```python
from build123d import *

# Parameters (mm, degrees)
F1_DEPTH = 63.5
F2_DEPTH = 25.4
F3_DEPTH = 12.7


with BuildPart() as f1:
    # F0 (on Front) → F1 (new body, symmetric)
    with BuildSketch(Plane.XZ):
        Polygon((41.275, -9.525), (41.275, 9.525), (22.225, 9.525), (-41.275, 9.525), (-41.275, -9.525), align=None)
    extrude(amount=F1_DEPTH, both=True)

    # F0 (on Front) → F2 (join, symmetric)
    with BuildSketch(Plane.XZ):
        with BuildLine():
            Line((22.225, 9.525), (41.275, 9.525))
            Line((41.275, 9.525), (41.275, 27.0002))
            ThreePointArc((41.275, 27.0002), (45.92468, 38.22552), (57.15, 42.8752))
            Line((57.15, 42.8752), (60.325, 42.8752))
            Line((60.325, 42.8752), (60.325, 61.9252))
            Line((60.325, 61.9252), (57.15, 61.9252))
            add(Edge.make_bspline(
                [(47.359648, 60.524887), (50.585981, 60.958071), (53.852213, 61.418514), (57.15, 61.9252)],
                knots=[103.904847, 103.904847, 103.904847, 103.904847, 111.504536, 111.504536, 111.504536, 111.504536], degree=3))
            ThreePointArc((47.359648, 60.524887), (29.206453, 47.950469), (22.225, 27.0002))
            Line((22.225, 27.0002), (22.225, 9.525))
        make_face()
        Polygon((60.325, 61.9252), (60.325, 42.8752), (60.325, 38.1), (111.125, 38.1), (111.125, 66.675), (60.325, 66.675), align=None)
    extrude(amount=F2_DEPTH, both=True)

    # F0 (on Front) → F3 (join, symmetric)
    with BuildSketch(Plane.XZ):
        Polygon((41.275, -9.525), (41.275, 9.525), (22.225, 9.525), (-41.275, 9.525), (-41.275, -9.525), align=None)
        with BuildLine():
            Line((22.225, 9.525), (41.275, 9.525))
            Line((41.275, 9.525), (41.275, 27.0002))
            ThreePointArc((41.275, 27.0002), (45.92468, 38.22552), (57.15, 42.8752))
            Line((57.15, 42.8752), (60.325, 42.8752))
            Line((60.325, 42.8752), (60.325, 61.9252))
            Line((60.325, 61.9252), (57.15, 61.9252))
            add(Edge.make_bspline(
                [(47.359648, 60.524887), (50.585981, 60.958071), (53.852213, 61.418514), (57.15, 61.9252)],
                knots=[103.904847, 103.904847, 103.904847, 103.904847, 111.504536, 111.504536, 111.504536, 111.504536], degree=3))
            ThreePointArc((47.359648, 60.524887), (29.206453, 47.950469), (22.225, 27.0002))
            Line((22.225, 27.0002), (22.225, 9.525))
        make_face()
        with BuildLine():
            Line((-41.275, 9.525), (22.225, 9.525))
            Line((22.225, 9.525), (22.225, 27.0002))
            ThreePointArc((22.225, 27.0002), (29.206453, 47.950469), (47.359648, 60.524887))
            add(Edge.make_bspline(
                [(-41.275, 9.525), (-33.40458, 53.775256), (3.24841, 54.602289), (47.359648, 60.524887)],
                knots=[0, 0, 0, 0, 103.904847, 103.904847, 103.904847, 103.904847], degree=3))
        make_face()
        with BuildLine():
            ThreePointArc((57.15, 61.9252), (52.205006, 61.573349), (47.359648, 60.524887))
            add(Edge.make_bspline(
                [(47.359648, 60.524887), (50.585981, 60.958071), (53.852213, 61.418514), (57.15, 61.9252)],
                knots=[103.904847, 103.904847, 103.904847, 103.904847, 111.504536, 111.504536, 111.504536, 111.504536], degree=3))
        make_face()
        Polygon((60.325, 61.9252), (60.325, 42.8752), (60.325, 38.1), (111.125, 38.1), (111.125, 66.675), (60.325, 66.675), align=None)
    extrude(amount=F3_DEPTH, both=True)


solid = f1.part
```
Read the model definition and answer for the solid it produces. Units are mm, in the model's axes. A direction names the side the tool comes from. Round coordinates to 2 decimals unless told otherwise and drop trailing zeros. Loops run counter-clockwise (first coordinate to the right, second up) from the corner with the lowest first, then second, coordinate; pieces in that order, holes last. Notation, with made-up numbers: (-26, 64) -> (-15, 64) arc R26 ccw to (-15, 87) -> close; hole circle Ø11 at (-13, -39.75). An arc over 180 degrees is marked (long way). One line per item, written item: value.
1) Consider L1, parallel to Z at x = 36, y = 43.5 (3 decimals); L2, parallel to X at y = -17.5, z = 25.5 (3 decimals); L3, parallel to Y at x = 19, z = 43. Determine where each line is inside the solid, lowest interval first. Write a range as [from, to].
Answer list:
L1: z = [-9.525, 9.525]
L2: x = [22.225, 41.275]
L3: y = [-12.7, 12.7]
2) A cutting plane is placed at B-B (x = 89). Determine the outline of the cut face in (y, z) (3 decimals).
Answer list:
outline: (-25.4, 38.1) -> (25.4, 38.1) -> (25.4, 66.675) -> (-25.4, 66.675) -> close
3) A cutting plane is placed at A-A (y = 45.5). Determine the outline of the cut face in (x, z) (3 decimals).
Answer list:
outline: (-41.275, -9.525) -> (41.275, -9.525) -> (41.275, 9.525) -> (-41.275, 9.525) -> close
4) The mould has two halves that part along X. Classify faces 1 (the face through (111.125, 0, 52)), 2 (the face through (60.325, 0, 41)), 3 (the face through (66, 25.4, 45)), 4 (the face through (29.396, 18.961, 48.201)): pulls with the +X half, pulls with the -X half, needs draft (parallel to the pull), parting line crosses it, or undercut.
Answer list:
face 1: pulls with the +X half
face 2: undercut
face 3: needs draft
face 4: pulls with the -X half
5) Flat-ended cylindrical pins translate along their axes: P1, Ø1, axis at x = 58.5, y = 6, coming from the +Z side; P2, Ø2.5, axis at x = 58, y = 11.5, coming from the -Z side; P3, Ø6, axis at x = 31.5, z = 48, coming from the -Y side; P4, Ø17, axis at x = 57.5, z = 27, coming from the +Y side. Find the tip coordinate at first contact, or state that the pin passes through.
Answer list:
P1: stops at z = 61.93
P2: stops at z = 42.87
P3: stops at y = -25.4
P4: passes through
6) For faces 5 (the face through (22.225, 19, 18)), 6 (the face through (41.275, -1, 4)), 7 (the face through (22.225, -19, 18)), 8 (the face through (60.325, 0, 64)), determine the directions among +Z, -Z, +X, -X, +Y, -Y from which every point of the face is accessible in a straight line to the end or side of a thin tool.
Answer list:
face 5: +Z, -X, +Y
face 6: -Z, +X, +Y, -Y
face 7: +Z, -X, -Y
face 8: +Z, -X, +Y, -Y
